The listing builds one solid part. Answer for the finished solid, in the listing's coordinates (mm). Round coordinates to 2 decimals unless told otherwise and drop trailing zeros. Write each loop counter-clockwise with the first axis right and the second up, starting at its lowest first coordinate (ties: lowest second). Pieces come first, ordered by that corner, then holes.
(1) A cutting plane is placed at D-D, the plane x = 0. Give the vertices of the cut face in (y, z), and give its area (3 significant figures).
(2) A cutting plane is placed at C-C, the plane y = 47. Give the vertices of the cut face in (x, z).
(3) The mould has two halves that part along X. Classify faces 1 (the face through (-6, 1, 0)), 2 (the face through (10.214, 55.671, -2.958)): +X half, -X half, draft (parallel to the pull), parting line (faces both ways), or undercut.
(4) A cutting plane is placed at B-B, the plane z = -4.9. Give the number of separate pieces and of enclosed holes in the cut face, and give its area (3 significant figures).
(5) A cutting plane is placed at A-A, the plane x = 133. Give the vertices of the cut face in (y, z).
(6) This flat-tipped pin is pushed along its axis until it touches: pin 1 Ø3 at (x, y) = (253.5, 35) entering from +Z. Where does it stop, or does it pass through?
(7) Find the intervals of material crossed by probe 1 along Y at (x, z) = (-23.5, -1.9); probe 2 along Y at (x, z) = (0, -2.8); probe 3 along Y at (x, z) = (369, -2.6), in increasing order.
from build123d import *

# Parameters (mm, degrees)
SKETCH1_W          = 788
SKETCH1_H          = 150
BASE_FLANGE1_DEPTH = 6
SKETCH2_W          = 50
SKETCH2_H          = 50
CUT_EXTRUDE1_DEPTH = 402.119682888
SKETCH3_R          = 19
SKETCH3_R_2        = 2.5
CUT_EXTRUDE2_DEPTH = 10
SKETCH4_R          = 3.25
CUT_EXTRUDE3_DEPTH = 10


# Sheet-metal steps are written as plain solids
with BuildPart() as part:
    # Sketch1 → Base-Flange1 (new body)
    with BuildSketch(Plane.XY):
        Rectangle(SKETCH1_W, SKETCH1_H)
    extrude(amount=-BASE_FLANGE1_DEPTH)

    # Sketch2 → Cut-Extrude1 (cut, through all)
    with BuildSketch(Plane.XY):
        with Locations((-125, 30)):
            Rectangle(SKETCH2_W, SKETCH2_H)
        with Locations((125, 30)):
            Rectangle(SKETCH2_W, SKETCH2_H)
    extrude(amount=-CUT_EXTRUDE1_DEPTH, mode=Mode.SUBTRACT)

    # Sketch3 → Cut-Extrude2 (cut)
    with BuildSketch(Plane.XY):
        with Locations((0, 39.65)):
            Circle(SKETCH3_R)
        with Locations((23.5, 63.15)):
            Circle(SKETCH3_R_2)
        with Locations((23.5, 16.15)):
            Circle(SKETCH3_R_2)
        with Locations((-23.5, 16.15)):
            Circle(SKETCH3_R_2)
        with Locations((-23.5, 63.15)):
            Circle(SKETCH3_R_2)
    extrude(amount=-CUT_EXTRUDE2_DEPTH, mode=Mode.SUBTRACT)

    # Sketch4 → Cut-Extrude3 (cut)
    with BuildSketch(Plane.XY):
        with Locations((369, -20)):
            Circle(SKETCH4_R)
        with Locations((-369, -20)):
            Circle(SKETCH4_R)
    extrude(amount=-CUT_EXTRUDE3_DEPTH, mode=Mode.SUBTRACT)


solid = part.part
Solutions:
1. outline: (-75, -6) - (20.65, -6) - (20.65, 0) - (-75, 0) - close; (58.65, -6) - (75, -6) - (75, 0) - (58.65, 0) - close
1. area: 672 mm2
2. outline: (-394, -6) - (-150, -6) - (-150, 0) - (-394, 0) - close; (-100, -6) - (-17.52, -6) - (-17.52, 0) - (-100, 0) - close; (17.52, -6) - (100, -6) - (100, 0) - (17.52, 0) - close; (150, -6) - (394, -6) - (394, 0) - (150, 0) - close
3. face 1: draft
3. face 2: undercut
4. separate pieces: 1
4. enclosed holes: 9
4. area: 112,000 mm2
5. outline: (-75, -6) - (5, -6) - (5, 0) - (-75, 0) - close; (55, -6) - (75, -6) - (75, 0) - (55, 0) - close
6. pin 1: stops at z = 0
7. probe 1: y = -75 to 13.65, 18.65 to 60.65, 65.65 to 75
7. probe 2: y = -75 to 20.65, 58.65 to 75
7. probe 3: y = -75 to -23.25, -16.75 to 75
